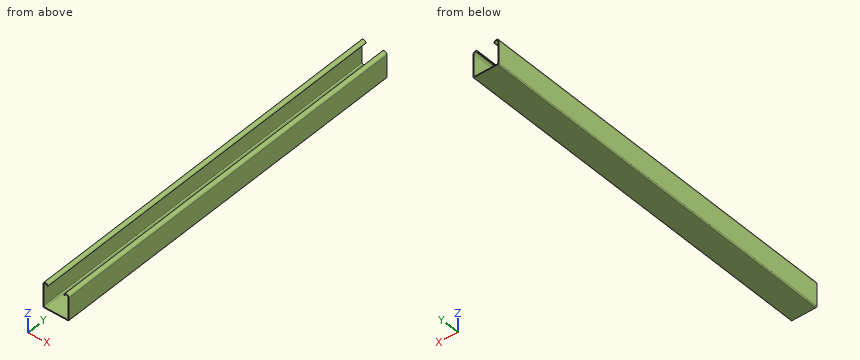
```python
from build123d import *

# Parameters (mm, degrees)
F1_DEPTH = 301.625
F2_R     = 1.5875
F3_R     = 0.635


with BuildPart() as f1:
    # F0 (on Front) → F1 (new body, symmetric)
    with BuildSketch(Plane.XZ):
        with BuildLine():
            Line((0, 37.3126), (0, 0))
            Line((0, 0), (41.275, 0))
            Line((41.275, 0), (41.275, 37.3126))
            ThreePointArc((41.275, 37.3126), (37.3126, 41.275), (33.3502, 37.3126))
            Line((33.3502, 37.3126), (34.9377, 37.3126))
            ThreePointArc((34.9377, 37.3126), (37.3126, 39.6875), (39.6875, 37.3126))
            Line((39.6875, 37.3126), (39.6875, 1.5875))
            Line((39.6875, 1.5875), (1.5875, 1.5875))
            Line((1.5875, 1.5875), (1.5875, 37.3126))
            ThreePointArc((1.5875, 37.3126), (3.9624, 39.6875), (6.3373, 37.3126))
            Line((6.3373, 37.3126), (7.9248, 37.3126))
            ThreePointArc((7.9248, 37.3126), (3.9624, 41.275), (0, 37.3126))
        make_face()
    extrude(amount=F1_DEPTH, both=True)

    # F2
    f2_edges = [f1.edges().sort_by_distance(p)[0] for p in [
        (0, 0, 0),
        (41.275, 0, 0),
        (39.6875, 0, 1.5875),
        (1.5875, 0, 1.5875),
    ]]
    fillet(f2_edges, radius=F2_R)

    # F3
    f3_edges = [f1.edges().sort_by_distance(p)[0] for p in [
        (6.3373, 0, 37.3126),
        (7.9248, 0, 37.3126),
        (33.3502, 0, 37.3126),
        (34.9377, 0, 37.3126),
    ]]
    fillet(f3_edges, radius=F3_R)


solid = f1.part
```
The model under review builds one solid part; all positions refer to its coordinate system, in mm. Coordinates: 2 decimals unless noted, no trailing zeros. Order: outer loops, then holes, each group sorted by start corner. A loop starts at its lowest first (then second) coordinate and runs counter-clockwise, first axis right, second up. Notation, with made-up numbers: (26, 33.5) -> (66, 33.5) arc R27 ccw to (66, 49.5) -> close; hole circle Ø6 at (15, 11.25). An arc over 180 degrees is marked (long way). Answer in a Markdown table with one row per item. Add a question column.
Item 1: To check wall thickness, follow probe 1 along X at (y, z) = (93, 20.5) (1 decimal); probe 2 along Z at (x, y) = (11.5, 77); probe 3 along X at (y, z) = (224.5, 37.5). State the ranges of each line that lie inside material, in increasing order.
Item 2: Clearance check with a flat-ended pin moving along its axis: pin 1 (12 mm diameter, centred on x = 7.5, y = 132.5, fed in from +Z) (3 decimals). State where the tip first meets the part, or that it passes through.
Item 3: We need section A-A on z = 19.5. Write out the cut boundary in (x, y) (1 decimal), plus the area to 3 significant figures.
Item 4: We need section C-C on x = 20. Write out the cut boundary in (y, z) (1 decimal).
Final values:
| question | item | result |
|---|---|---|
| 1 | probe 1 | x = 0 to 1.6, 39.7 to 41.3 |
| 1 | probe 2 | z = 0 to 1.59 |
| 1 | probe 3 | x = 0 to 1.59, 6.45 to 7.68, 33.6 to 34.82, 39.68 to 41.27 |
| 2 | pin 1 | stops at z = 41.275 |
| 3 | outline | (0, -301.6) -> (1.6, -301.6) -> (1.6, 301.6) -> (0, 301.6) -> close; (39.7, -301.6) -> (41.3, -301.6) -> (41.3, 301.6) -> (39.7, 301.6) -> close |
| 3 | area | 1,920 mm2 |
| 4 | outline | (-301.6, 0) -> (301.6, 0) -> (301.6, 1.6) -> (-301.6, 1.6) -> close |
